The model under review builds one solid part; all positions refer to its coordinate system, in mm. A direction names the side the tool comes from. Coordinates: 2 decimals unless noted, no trailing zeros. Write each loop counter-clockwise with the first axis right and the second up, starting at its lowest first coordinate (ties: lowest second). Pieces come first, ordered by that corner, then holes. Notation, with made-up numbers: (75.25, -39.5) - (98.25, -39.5) arc R29 cw to (98.25, -0.5) - close; hole circle Ø3 at (0.5, 5.25). An arc over 180 degrees is marked (long way). Answer as CSV lines item,"result". Start each with the question number.
```python
from build123d import *

# Parameters (mm, degrees)
F0_W         = 14
F0_H         = 10
F1_DEPTH     = 1.5
F2_W         = 9
F2_H         = 7
F3_DEPTH     = 25
F4_W         = 12
F4_H         = 10
F4_W_2       = 9
F4_H_2       = 7
F5_DEPTH     = 29
F6_W         = 12
F6_H         = 10
F7_DEPTH     = 0.5
F8_R         = 3.5
F9_DEPTH     = 25
F10_W        = 2.1
F10_H        = 2.1
F11_DEPTH    = 11
F12_W        = 10
F12_H        = 6.5
F13_DEPTH    = 1.5
F14_W        = 10
F14_H        = 6.3
F15_DEPTH    = 1.5
F16_T1_DEPTH = 9


# Not quite as in the source:
# - a fillet or chamfer that OpenCascade refuses, or shapes differently, is made with other operations: its cross-section is extruded or revolved along the edge and cut away or added


with BuildPart() as f1:
    # F0 (on Top) → F1 (new body)
    with BuildSketch(Plane.XY):
        with Locations((7, 5)):
            Rectangle(F0_W, F0_H)
    extrude(amount=F1_DEPTH)

    # F2 (on face) → F3 (cut)
    with BuildSketch(Plane.XY.offset(1.5)):
        with Locations((6.4, 5)):
            Rectangle(F2_W, F2_H)
    extrude(amount=-F3_DEPTH, mode=Mode.SUBTRACT)

    # F4 (on face) → F5 (join)
    with BuildSketch(Plane.XY.offset(1.5)):
        with Locations((6.4, 5)):
            Rectangle(F4_W, F4_H)
        with Locations((6.4, 5)):
            Rectangle(F4_W_2, F4_H_2, mode=Mode.SUBTRACT)
    extrude(amount=F5_DEPTH)

    # F6 (on face) → F7 (join)
    with BuildSketch(Plane.XY.offset(30.5)):
        with Locations((6.4, 5)):
            Rectangle(F6_W, F6_H)
    extrude(amount=F7_DEPTH)

    # F8 (on face) → F9 (cut)
    with BuildSketch(Plane.YZ.offset(12.4)):
        with Locations((4.7, 28.0150376887)):
            Circle(F8_R)
    extrude(amount=-F9_DEPTH, mode=Mode.SUBTRACT)

    # F10 (on face) → F11 (cut)
    with BuildSketch(Plane(origin=(0, 0, 0), x_dir=(1, 0, 0), z_dir=(0, 0, -1))):
        with Locations((11.95, -4.75)):
            Rectangle(F10_W, F10_H)
    extrude(amount=-F11_DEPTH, mode=Mode.SUBTRACT)

    # F12 (on face) → F13 (cut)
    with BuildSketch(Plane(origin=(0.4, 0, 0), x_dir=(0, -1, 0), z_dir=(-1, 0, 0))):
        with Locations((-5, 4.75)):
            Rectangle(F12_W, F12_H)
    extrude(amount=-F13_DEPTH, mode=Mode.SUBTRACT)

    # F14 (on face) → F15 (cut)
    with BuildSketch(Plane.YZ.offset(12.4)):
        with Locations((5, 4.65)):
            Rectangle(F14_W, F14_H)
    extrude(amount=-F15_DEPTH, mode=Mode.SUBTRACT)

    # F16: fillet of radius 5 on 2 edges, made by hand

    # F16_s2 → F16_t1 (cut)
    with BuildSketch(Plane.YZ.offset(1.9)):
        with BuildLine():
            ThreePointArc((8.5, 5), (9.9644660941, 1.4644660941), (13.5, 0))
            Line((13.5, 0), (13.5, -0.1))
            Line((13.5, -0.1), (8.4, -0.1))
            Line((8.4, -0.1), (8.4, 5))
            Line((8.4, 5), (8.5, 5))
        make_face()
        with BuildLine():
            ThreePointArc((1.5, 5), (0.0355339059, 1.4644660941), (-3.5, 0))
            Line((-3.5, 0), (-3.5, -0.1))
            Line((-3.5, -0.1), (1.6, -0.1))
            Line((1.6, -0.1), (1.6, 5))
            Line((1.6, 5), (1.5, 5))
        make_face()
    extrude(amount=F16_T1_DEPTH, mode=Mode.SUBTRACT)


solid = f1.part
```
(1) Add section C-C on x = 4.5. Give the boundary of the cut face in (y, z).
(2) For faces 5 (the flat face through (1.9, 5, 17)), 6 (the flat face through (10.9, 9, 5)), 7 (the flat face through (1.9, 9, 6)), 8 (the flat face through (12, 3.7, 9)), list the 3-axis set-ups (+Z, -Z, +X, -X, +Y, -Y) from which the entire face can be reached by the end or side of a thin tool; tool diameter is ignored.
(3) Add section D-D on z = 18. Give the boundary of the cut face in (x, y).
(4) Add section B-B on y = 4.7. Give the boundary of the cut face in (x, z), then the cut area to 3 significant figures.
(5) Wall thickness on line 1 (Y direction, x = 9, z = 23); line 2 (X direction, y = 8, z = 11.5); line 3 (Z direction, x = 1.5, y = 1): over which ranges is each line inside the solid? List them lowest first.
(6) The part is to be moulded in two halves that separate along Y. For faces 1 (the cylindrical face through (6.484, 1.265, 28.689)), 2 (the flat face through (6, 1.5, 30)), 3 (the flat face through (7, 0, 15)), 4 (the flat face through (13.5, 5.1, 0)), say which applies: released by +Y, released by -Y, zero draft, split by the parting line, or undercut.
(7) Add section A-A on x = 11.75. Give the boundary of the cut face in (y, z), then the cut area to 3 significant figures.
(8) For pin 1 (1.5 mm diameter, centred on x = 12.5, y = 5, fed in from +Z); pin 2 (1 mm diameter, centred on y = 3, z = 18.5, fed in from +X); pin 3 (1.2 mm diameter, centred on y = 0.5, z = 4.5, fed in from +X); pin 4 (1.6 mm diameter, centred on x = 12, y = 2, fed in from -Z), all flat-tipped, find the tip position at first contact; note any pin that passes through.
Reported:
1,outline,"(0, 1.43) arc R5 ccw to (1.5, 5) - (1.5, 26.6) arc R3.5 cw to (1.5, 29.43) - (1.5, 30.5) - (2.24, 30.5) arc R3.5 cw to (2.87, 31) - (0, 31) - close; (6.53, 31) arc R3.5 cw to (7.16, 30.5) - (8.5, 30.5) - (8.5, 5) arc R5 ccw to (10, 1.43) - (10, 31) - close"
2,face 5,"-Z"
2,face 6,"+X, +Y, -Y"
2,face 7,"-X, +Y, -Y"
2,face 8,"-Z, +X"
3,outline,"(0.4, 0) - (12.4, 0) - (12.4, 10) - (0.4, 10) - close; hole (1.9, 1.5) - (10.9, 1.5) - (10.9, 8.5) - (1.9, 8.5) - close"
4,outline,"(0, 0) - (1.9, 0) - (1.9, 1.5) - (0, 1.5) - close; (0.4, 8) - (1.9, 8) - (1.9, 24.52) - (0.4, 24.52) - close; (10.9, 11) - (12.4, 11) - (12.4, 24.52) - (10.9, 24.52) - close; (13, 0) - (14, 0) - (14, 1.5) - (13, 1.5) - close"
4,area,"49.4 mm²"
5,line 1,"0 to 1.5, 8.5 to 10"
5,line 2,"0.4 to 1.9, 10.9 to 12.4"
5,line 3,"0 to 1.5, 8 to 31"
6,face 1,"undercut"
6,face 2,"undercut"
6,face 3,"released by -Y"
6,face 4,"zero draft"
7,outline,"(0, 0) - (3.7, 0) - (3.7, 1.5) - (0, 1.5) - close; (0, 7.8) - (3.7, 7.8) - (3.7, 11) - (5.8, 11) - (5.8, 7.8) - (10, 7.8) - (10, 31) - (6.53, 31) arc R3.5 cw (long way) to (2.87, 31) - (0, 31) - close; (5.8, 0) - (10, 0) - (10, 1.5) - (5.8, 1.5) - close"
7,area,"200 mm²"
8,pin 1,"z = 24.67"
8,pin 2,"x = 12.4"
8,pin 3,"x = 10.9"
8,pin 4,"z = 0"
